Here's how the part is built. I have some questions about the finished solid (model axes, mm). Face numbers are marked on the shaded views. Give positions to 0.01 mm unless a question says otherwise; leave off trailing zeros. Write each loop counter-clockwise with the first axis right and the second up, starting at its lowest first coordinate (ties: lowest second). Pieces come first, ordered by that corner, then holes. Notation, with made-up numbers: (53, 7) -> (110, 7) arc R17 cw to (110, 32) -> close; hole circle Ø4 at (37, -0.5). An arc over 180 degrees is marked (long way). Return JSON: item names as keys, results as strings.
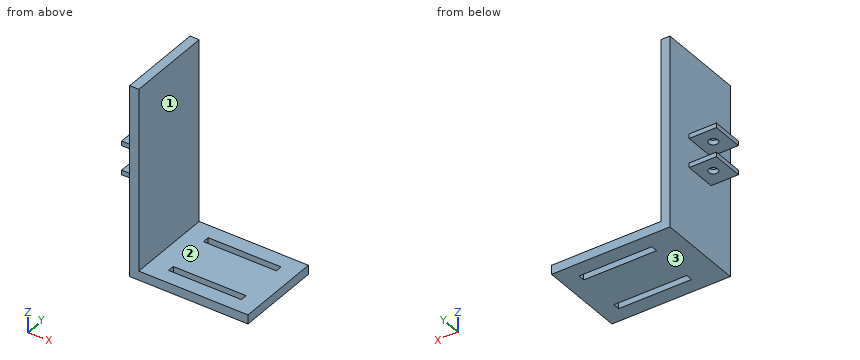
Autodesk Inventor part; units mm, degrees
ref_plane "YZ Plane" through (0, 0, 0) normal (1, 0, 0) x (0, 1, 0)
ref_plane "XZ Plane" through (0, 0, 0) normal (0, 1, 0) x (-1, 0, 0)
ref_plane "XY Plane" through (0, 0, 0) normal (0, 0, 1) x (1, 0, 0)
sketch "Sketch1" plane through (0, 0, 0) normal (0, 0, 1) x (1, 0, 0)
  line L0 (0, 0) -> (165.1, 0)
  line L1 (165.1, 0) -> (165.1, 120.65)
  line L2 (165.1, 120.65) -> (0, 120.65)
  line L3 (0, 120.65) -> (0, 0)
  dimension "d0" = 165.1
  dimension "d1" = 120.65
extrude "Extrusion1" add sketch "Sketch1" against normal blind 12.7
sketch "Sketch2" plane through (0, 0, 0) normal (0, 0, 1) x (1, 0, 0)
  line L0 (165.1, 0) -> (0, 0)
  line L1 (0, 120.65) -> (165.1, 120.65)
  line L2 (0, 0) -> (12.7, 0)
  line L3 (12.7, 0) -> (12.7, 120.65)
  line L4 (12.7, 120.65) -> (0, 120.65)
  line L5 (0, 120.65) -> (0, 0)
  dimension "d4" = 12.7
extrude "Extrusion2" add sketch "Sketch2" along normal blind 254
sketch "Sketch5" plane through (0, 0, 0) normal (0, 0, 1) x (1, 0, 0)
  point P0 (0, 0)
sketch "Sketch7" plane through (0, 0, 0) normal (0, 0, 1) x (1, 0, 0)
  line L0 (165.1, 120.65) -> (165.1, 0)
  line L1 (165.1, 60.325) -> (0, 60.325)
  line L2 (0, 0) -> (0, 120.65)
  line L3 (39.7226, 30.1625) -> (141.3226, 30.1625)
  line L4 (141.3226, 30.1625) -> (141.3226, 20.6375)
  line L5 (141.3226, 20.6375) -> (39.7226, 20.6375)
  line L6 (39.7226, 20.6375) -> (39.7226, 30.1625)
  line L7 (39.7226, 90.4875) -> (141.3226, 90.4875)
  line L8 (141.3226, 90.4875) -> (141.3226, 100.0125)
  line L9 (141.3226, 100.0125) -> (39.7226, 100.0125)
  line L10 (39.7226, 100.0125) -> (39.7226, 90.4875)
  point P0 (118.0813, 25.4)
  point P1 (118.0813, 95.25)
  dimension "d20" = 101.6
  dimension "d21" = 9.525
  dimension "d33" = 4.7625
  dimension "d34" = 4.7625
hole "Hole1" [suppressed]
extrude "Extrusion7" cut sketch "Sketch7" against normal blind 25.4
sketch "Sketch8" plane through (0, 0, -12.7) normal (-1, 0, 0) x (0, 0, 1)
  line L0 (266.7, 120.65) -> (266.7, 0)
  line L1 (266.7, 60.325) -> (0, 60.325)
  line L2 (0, 0) -> (0, 120.65)
  line L3 (128.4341, 144.8996) -> (128.4341, -24.2496)
  line L4 (145.5791, 60.325) -> (145.5791, 38.354)
  line L5 (145.5791, 60.325) -> (145.5791, 82.296)
  line L6 (111.2891, 60.325) -> (111.2891, 38.354)
  line L7 (111.2891, 60.325) -> (111.2891, 82.296)
  line L8 (145.5791, 82.296) -> (151.9291, 82.296)
  line L9 (151.9291, 82.296) -> (151.9291, 38.354)
  line L10 (151.9291, 38.354) -> (145.5791, 38.354)
  line L11 (145.5791, 38.354) -> (145.5791, 82.296)
  line L12 (111.2891, 82.296) -> (104.9391, 82.296)
  line L13 (104.9391, 82.296) -> (104.9391, 38.354)
  line L14 (104.9391, 38.354) -> (111.2891, 38.354)
  line L15 (111.2891, 38.354) -> (111.2891, 82.296)
  point P0 (12.7, 0)
  dimension "d35" = 17.145
  dimension "d36" = 21.971
  dimension "d37" = 21.971
  dimension "d38" = 6.35
  dimension "d39" = 6.35
extrude "Extrusion8" add sketch "Sketch8" along normal blind 38.1
sketch "Sketch9" plane through (0, 38.354, 139.2291) normal (0, 0, 1) x (1, 0, 0)
  line L0 (0, 82.296) -> (0, -38.354)
  circle A0 centre (-19.05, 22.7915) radius 6.35
  point P0 (0, 22.7915)
  dimension "d42" = 19.05
  dimension "d43" = 12.7
extrude "Extrusion9" cut sketch "Sketch9" against normal blind 50.8
properties part number "LucasCharles part11 final" material "Stainless Steel, Austenitic"
1. For pin 1 Ø1.9 at (x, z) = (-13.5, 96) entering from +Y; pin 2 Ø8 at (y, z) = (87.5, 65) entering from -X; pin 3 Ø5 at (y, z) = (54.5, 177) entering from +X, each with a flat end and sliding along its axis, tell me the tip position at first contact or that it passes through.
Taken from the geometry:
{"pin 1": "stops at y = 82.3", "pin 2": "stops at x = 0", "pin 3": "stops at x = 12.7"}
2. Suppose I cut it at C-C, the plane y = 106. List the corners of the cut face in (x, z) for me.
Taken from the geometry:
{"outline": "(0, -12.7) -> (165.1, -12.7) -> (165.1, 0) -> (12.7, 0) -> (12.7, 254) -> (0, 254) -> close"}
3. Suppose I cut it at A-A, the plane x = -19.05. List the corners of the cut face in (y, z) for me, and give its area (3 significant figures).
Taken from the geometry:
{"outline": "(38.35, 92.24) -> (54.8, 92.24) -> (54.8, 98.59) -> (38.35, 98.59) -> close; (38.35, 132.88) -> (54.8, 132.88) -> (54.8, 139.23) -> (38.35, 139.23) -> close; (67.5, 92.24) -> (82.3, 92.24) -> (82.3, 98.59) -> (67.5, 98.59) -> close; (67.5, 132.88) -> (82.3, 132.88) -> (82.3, 139.23) -> (67.5, 139.23) -> close", "area": "397 mm²"}
4. If I drill on line 1 (Y direction, x = -19.05, z = 95.5); line 2 (X direction, y = 67.5, z = 81.5); line 3 (Z direction, x = 126, y = 76.5), over which ranges is the centre line in solid material (lowest first)? Write a range as [from, to].
Taken from the geometry:
{"line 1": "y = [38.35, 54.8], [67.5, 82.3]", "line 2": "x = [0, 12.7]", "line 3": "z = [-12.7, 0]"}
5. Suppose I cut it at B-B, the plane x = 104.5. List the corners of the cut face in (y, z) for me.
Taken from the geometry:
{"outline": "(0, -12.7) -> (20.64, -12.7) -> (20.64, 0) -> (0, 0) -> close; (30.16, -12.7) -> (90.49, -12.7) -> (90.49, 0) -> (30.16, 0) -> close; (100.01, -12.7) -> (120.65, -12.7) -> (120.65, 0) -> (100.01, 0) -> close"}
6. Suppose I cut it at D-D, the plane z = 222. List the corners of the cut face in (x, y) for me.
Taken from the geometry:
{"outline": "(0, 0) -> (12.7, 0) -> (12.7, 120.65) -> (0, 120.65) -> close"}
7. If we mould it in two halves opening along Z, with no side actions, what happens to the marked faces 1, 2 and 3? For each: released by +Z, released by -Z, zero draft, split by the parting line, or undercut.
Taken from the geometry:
{"face 1": "zero draft", "face 2": "released by +Z", "face 3": "released by -Z"}
